```python
from build123d import *

# Parameters (mm, degrees)
F0_R     = 20
F0_R_2   = 3.9
F1_DEPTH = 3
F2_W     = 10
F2_H     = 2.98
F3_DEPTH = 25


with BuildPart() as f1:
    # F0 (on Front) → F1 (new body)
    with BuildSketch(Plane.XZ):
        Circle(F0_R)
        Circle(F0_R_2, mode=Mode.SUBTRACT)
    extrude(amount=F1_DEPTH)

    # F2 (on face) → F3 (cut)
    with BuildSketch(Plane.XZ.offset(3)):
        with Locations((0, -15)):
            Rectangle(F2_W, F2_H)
        Polygon((14.200003, -2.424873), (9.200003, -11.085127), (11.780759, -12.575127), (16.780759, -3.914873), align=None)
        Polygon((9.200003, 11.085127), (14.200003, 2.424873), (16.780759, 3.914873), (11.780759, 12.575127), align=None)
        with Locations((0, 15)):
            Rectangle(F2_W, F2_H)
        Polygon((-14.200003, 2.424873), (-9.200003, 11.085127), (-11.780759, 12.575127), (-16.780759, 3.914873), align=None)
        Polygon((-9.200003, -11.085127), (-14.200003, -2.424873), (-16.780759, -3.914873), (-11.780759, -12.575127), align=None)
    extrude(amount=-F3_DEPTH, mode=Mode.SUBTRACT)


solid = f1.part
```
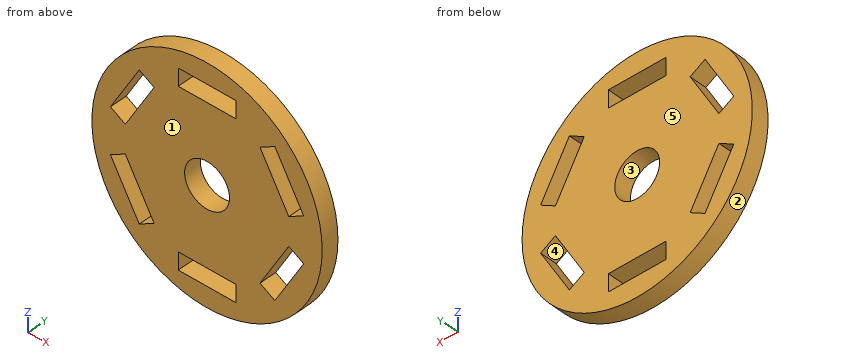
Verification items for the finished model (mm, model axes). Face numbers are marked on the shaded views. A direction names the side the tool comes from. Give positions to 0.01 mm unless a question says otherwise; leave off trailing zeros. Loops run counter-clockwise (first coordinate to the right, second up) from the corner with the lowest first, then second, coordinate; pieces in that order, holes last. Notation, with made-up numbers: M -27.5,16.25 L -4.5,16.25 A30 cw -4.5,50.25 Z; hole C 52,31.25 d11. An arc over 180 degrees is marked long. Return JSON: item names as keys, results as strings.
1) Tool access check on the marked faces 4 and 5. Record the directions out of +Z, -Z, +X, -X, +Y, -Y that give a thin tool (end or side, any length) a straight path to the whole face; none if there is none.
Findings:
{"face 4": "+Y, -Y", "face 5": "+Z, -Z, +X, -X, +Y"}
2) Material ranges on L1, parallel to Z at x = 0, y = -0.9; L2, parallel to Z at x = -14.5, y = -0.2; L3, parallel to X at y = -2.55, z = 8, recorded low to high. Write a range as [from, to].
Findings:
{"L1": "z = [-20, -16.49], [-13.51, -3.9], [3.9, 13.51], [16.49, 20]", "L2": "z = [-13.77, -7.87], [-2.6, 2.6], [7.87, 13.77]", "L3": "x = [-18.33, -14.42], [-10.98, 10.98], [14.42, 18.33]"}
3) Mould release check, pull along Z, two halves, no side actions. Record for the marked faces 1, 2 and 3: released by +Z, released by -Z, zero draft, split by the parting line, or undercut.
Findings:
{"face 1": "zero draft", "face 2": "split by the parting line", "face 3": "undercut"}
4) Gauge pin test, flat ends, axial feed: P1, Ø0.9, axis at y = -1, z = -15.5, coming from the +X side; P2, Ø1.5, axis at x = 2.5, y = -2, coming from the +Z side; P3, Ø1.5, axis at x = -1, y = -1, coming from the -Z side. Record the tip position at first contact, or that the pin passes through.
Findings:
{"P1": "stops at x = 13.17", "P2": "stops at z = 19.92", "P3": "stops at z = -20"}
5) Section check C-C, the plane y = -2. Enter the section's corners in (x, z), and give its area (3 significant figures).
Findings:
{"outline": "C 0,0 d40; hole M -16.78,-3.91 L -11.78,-12.58 L -9.2,-11.09 L -14.2,-2.42 Z; hole M -16.78,3.91 L -14.2,2.42 L -9.2,11.09 L -11.78,12.58 Z; hole M -5,-16.49 L 5,-16.49 L 5,-13.51 L -5,-13.51 Z; hole M -5,13.51 L 5,13.51 L 5,16.49 L -5,16.49 Z; hole C 0,0 d7.8; hole M 9.2,-11.09 L 11.78,-12.58 L 16.78,-3.91 L 14.2,-2.42 Z; hole M 9.2,11.09 L 14.2,2.42 L 16.78,3.91 L 11.78,12.58 Z", "area": "1,030 mm2"}
6) Section check A-A, the plane x = 0. Enter the section's corners in (y, z).
Findings:
{"outline": "M -3,-20 L 0,-20 L 0,-16.49 L -3,-16.49 Z; M -3,-13.51 L 0,-13.51 L 0,-3.9 L -3,-3.9 Z; M -3,3.9 L 0,3.9 L 0,13.51 L -3,13.51 Z; M -3,16.49 L 0,16.49 L 0,20 L -3,20 Z"}
7) Section check B-B, the plane z = 0. Enter the section's corners in (x, y).
Findings:
{"outline": "M -20,-3 L -3.9,-3 L -3.9,0 L -20,0 Z; M 3.9,-3 L 20,-3 L 20,0 L 3.9,0 Z"}
